Autodesk Inventor part; units mm, degrees
ref_plane "YZ Plane" through (0, 0, 0) normal (1, 0, 0) x (0, 1, 0)
ref_plane "XZ Plane" through (0, 0, 0) normal (0, 1, 0) x (-1, 0, 0)
ref_plane "XY Plane" through (0, 0, 0) normal (0, 0, 1) x (1, 0, 0)
sketch "Sketch1" plane through (0, 0, 0) normal (0, 1, 0) x (-1, 0, 0)
  line L0 (0, 0) -> (200, 0)
  line L1 (200, 0) -> (200, -150)
  line L2 (200, -150) -> (0, -150)
  line L3 (0, -150) -> (0, 0)
  dimension "d0" = 200
  dimension "d1" = 150
extrude "Extrusion1" add sketch "Sketch1" along normal blind 2
sketch "Sketch2" plane through (0, 0, 0) normal (0, -1, 0) x (1, 0, 0)
  line L0 (-200, 0) -> (0, 0)
  line L1 (-200, 0) -> (-198, 0)
  line L2 (-198, 0) -> (-198, -2)
  line L3 (-198, -2) -> (-2, -2)
  line L4 (-2, -2) -> (-2, -148)
  line L5 (-2, -148) -> (0, -148)
  line L6 (0, 0) -> (0, -150)
  dimension "d4" = 2
  dimension "d5" = 2
  dimension "d6" = 196
  dimension "d7" = 146
extrude "Extrusion2" add sketch "Sketch2" along normal blind 102
sketch "Sketch3" plane through (-200, 2, 0) normal (0, 0, 1) x (1, 0, 0)
  line L0 (0, -2) -> (2, -2)
  line L1 (2, -2) -> (6.5, -2)
  line L2 (198, -2) -> (2, -2)
  line L3 (6.5, -2) -> (6.5, -5.5)
  circle A0 centre (6.5, -5.5) radius 1
  line L4 (2, -104) -> (198, -104)
  line L5 (2, -104) -> (6.5, -104)
  line L6 (6.5, -104) -> (6.5, -99.5)
  circle A1 centre (6.5, -99.5) radius 1
  line L7 (200, -104) -> (2, -104)
  line L8 (200, -104) -> (194.5, -104)
  line L9 (194.5, -104) -> (194.5, -99.5)
  circle A2 centre (194.5, -99.5) radius 1
  point P0 (200, -2)
  dimension "d10" = 4.5
  dimension "d11" = 3.5
  dimension "d12" = 2
  dimension "d13" = 4.5
  dimension "d14" = 4.5
  dimension "d15" = 5.5
extrude "Extrusion3" cut sketch "Sketch3" against normal blind 10
sketch "Sketch4" plane through (0, 2, 0) normal (1, 0, 0) x (0, 0, -1)
  line L0 (148, -2) -> (148, -104)
  line L1 (148, -2) -> (143.5, -2)
  line L2 (150, -2) -> (0, -2)
  line L3 (143.5, -2) -> (143.5, -5.5)
  line L4 (148, -104) -> (143.5, -104)
  line L5 (143.5, -104) -> (143.5, -99.5)
  line L6 (143.5, -99.5) -> (148, -99.5)
  line L7 (148, -99.5) -> (148, -104)
  circle A0 centre (143.5, -99.5) radius 1
  circle A1 centre (143.5, -5.5) radius 1
  dimension "d18" = 4.5
  dimension "d19" = 3.5
  dimension "d20" = 4.5
  dimension "d21" = 4.5
  dimension "d22" = 2
extrude "Extrusion4" cut sketch "Sketch4" against normal blind 10 contours A1 | A0 L5 L6 | L6 L5 A0
sketch "Sketch5" plane through (0, 0, 0) normal (0, -1, 0) x (1, 0, 0)
  line L0 (-2, -148) -> (-2, -2)
  line L1 (-2, -75) -> (-172, -75)
  line L2 (-200, -150) -> (-200, 0)
  line L3 (-172, -75) -> (-174, -75)
  line L4 (-172, -75) -> (-172, -2)
  line L5 (-2, -2) -> (-198, -2)
  line L6 (0, -150) -> (-200, -150)
  line L7 (-172, -2) -> (-2, -2)
  line L8 (-2, -2) -> (-2, -150)
  line L9 (-2, -150) -> (-172, -150)
  line L10 (-172, -150) -> (-172, -2)
  line L11 (-200, 0) -> (0, 0)
  line L12 (-174, 0) -> (-2, 0)
  line L13 (-2, 0) -> (-2, -150)
  line L14 (-2, -150) -> (-174, -150)
  line L15 (-174, -150) -> (-174, 0)
  dimension "d28" = 170
  dimension "d29" = 2
sketch "Sketch6" plane through (-2, 0, -2) normal (0, 0, -1) x (-1, 0, 0)
  point P0 (-2, 0)
extrude "Extrusion5" cut sketch "Sketch5" along normal mid plane 1000 contours L15 L6 L2 L11
sketch "Sketch7" plane through (0, 0, 0) normal (0, -1, 0) x (1, 0, 0)
  line L0 (-174, -2) -> (-2, -2)
  line L1 (-174, -2) -> (-172, -2)
  line L2 (-172, -2) -> (-172, 0)
  line L3 (-174, 0) -> (0, 0)
  line L4 (-174, 0) -> (-172, 0)
  line L5 (-174, 0) -> (-174, -2)
  dimension "d32" = 2
extrude "Extrusion6" cut sketch "Sketch7" along normal blind 1000
sketch "Sketch9" plane through (0, 0, 0) normal (0, -1, 0) x (1, 0, 0)
  line L0 (0, -148) -> (0, 0)
  line L1 (0, -74) -> (-182, -74)
  line L2 (-174, 0) -> (-174, -150)
  line L3 (-174, 0) -> (-182, 0)
  line L4 (-182, 0) -> (-182, -150)
  line L5 (-182, -150) -> (-174, -150)
  line L6 (-174, -150) -> (-174, 0)
  dimension "d44" = 182
extrude "Extrusion8" add sketch "Sketch9" against normal blind 2
sketch "Sketch10" plane through (-2, -102, -2) normal (0, 0, -1) x (-1, 0, 0)
  line L0 (180, 102) -> (-2, 102)
  line L1 (180, 102) -> (178, 102)
  line L2 (170, 102) -> (170, 0)
  line L3 (178, 102) -> (170, 102)
  line L4 (170, 102) -> (170, 0)
  line L5 (170, 0) -> (178, 0)
  line L6 (178, 0) -> (178, 102)
  dimension "d47" = 2
extrude "Extrusion9" add sketch "Sketch10" against normal blind 2
sketch "Sketch11" plane through (-2, -102, -2) normal (0, 0, -1) x (-1, 0, 0)
  line L0 (0, 102) -> (178, 102)
  line L1 (178, 102) -> (178, 98.5)
  line L2 (178, 0) -> (178, 102)
  line L3 (178, 98.5) -> (173.5, 98.5)
  line L4 (178, 0) -> (0, 0)
  line L5 (178, 0) -> (173.5, 0)
  line L6 (173.5, 0) -> (173.5, 4.5)
  circle A0 centre (173.5, 98.5) radius 1
  circle A1 centre (173.5, 4.5) radius 1
  point P0 (-2, 102)
  dimension "d50" = 3.5
  dimension "d51" = 4.5
  dimension "d52" = 4.5
  dimension "d53" = 2
extrude "Extrusion10" cut sketch "Sketch11" against normal blind 2
properties part number "kevnat part2"
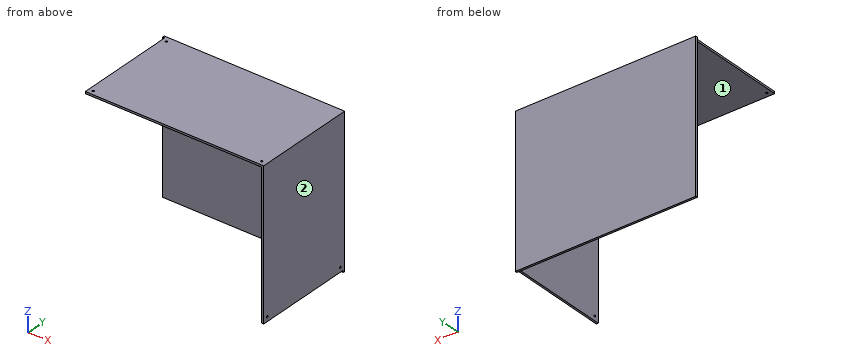
CAD build for the part. Positions are in the model's coordinates, mm. Face numbers are marked on the shaded views. A direction names the side the tool comes from. Round coordinates to 2 decimals unless told otherwise and drop trailing zeros. Order: outer loops, then holes, each group sorted by start corner. A loop starts at its lowest first (then second) coordinate and runs counter-clockwise, first axis right, second up. Notation, with made-up numbers: (-3, -32.75) -> (32, -32.75) arc R6 cw to (32, -27.75) -> close; hole circle Ø7 at (-33, 17). An arc over 180 degrees is marked (long way). One line per question, with ' | ' between items.
Q1. Probe probe 1 along Y at (x, z) = (-0.65, -143.5); probe 2 along X at (y, z) = (-97.5, -1.15); probe 3 along Z at (x, y) = (-0.7, -97.5). List the from-to ranges inside material, lowest first.
Completed:
probe 1: y = -102 to -98.5, -96.5 to -4.5, -2.5 to 2 | probe 2: x = -180 to -176.5, -174.5 to -6.5, -4.5 to 0 | probe 3: z = -148 to -144.5, -142.5 to 0
Q2. Slice it at B-B (y = -74.5). Write the cut outline in (x, z).
Completed:
outline: (-180, -2) -> (-2, -2) -> (-2, -148) -> (0, -148) -> (0, 0) -> (-180, 0) -> close
Q3. Slice it at A-A (z = -126.5). Write the cut outline in (x, y), then the cut area to 3 significant figures.
Completed:
outline: (-182, 0) -> (-2, 0) -> (-2, -102) -> (0, -102) -> (0, 2) -> (-182, 2) -> close | area: 568 mm^2
Q4. Which spindle directions (+Z, -Z, +X, -X, +Y, -Y) get a long thin tool onto all of the face, cutting with end or side? Do the marked faces 1 and 2. Say none if no direction does.
Completed:
face 1: -Z, -X, -Y | face 2: +Z, -Z, +X, +Y, -Y
Q5. Drop flat-ended pins along their axis: pin 1 (5 mm diameter, centred on x = -52, y = -81, fed in from -Z); pin 2 (4 mm diameter, centred on y = -15, z = -88, fed in from -X); pin 3 (1.6 mm diameter, centred on x = -5.5, y = -97.5, fed in from +Z); pin 4 (0.6 mm diameter, centred on y = -65, z = -0.5, fed in from -X). Give the stop position or say it passes through.
Completed:
pin 1: stops at z = -2 | pin 2: stops at x = -2 | pin 3: passes through | pin 4: stops at x = -180
